Here's how the part is built. I have some questions about the finished solid (model axes, mm). A direction names the side the tool comes from. Coordinates: 2 decimals unless noted, no trailing zeros. Loops run counter-clockwise (first coordinate to the right, second up) from the corner with the lowest first, then second, coordinate; pieces in that order, holes last. Notation, with made-up numbers: (-27, -20.5) -> (-14, -20.5) arc R35 cw to (-14, 13.5) -> close; hole circle Ø1 at (-10.5, -10.5). An arc over 180 degrees is marked (long way). Answer as a JSON object with one key per item and string values. Group by question number.
1) Which directions (+Z, -Z, +X, -X, +Y, -Y) give clear straight access to the entire face, cutting with the end or side of a thin tool? Please do faces 1 (the flat face through (9.413, -7.048, 2.465)), 2 (the flat face through (3.94, 4.16, 5.07)), 3 (the flat face through (4.1, -6, 2.5)).
2) I want a section at A-A (y = 3.75). Write out the boundary of the cut face in (x, z), then the cut area to 3 significant figures.
3) If we mould it in two halves opening along Z, with no side actions, what happens to faces 4 (the cylindrical face through (4.264, -4.222, 6.479)), 5 (the cylindrical face through (5.99, 5.3, 2.46)), 6 (the flat face through (2, -4, 10))? For each: +Z half, -Z half, draft (parallel to the pull), parting line (faces both ways), or undercut.
4) I need wall thicknesses on probe 1 along Y at (x, z) = (3, 7.75); probe 2 along Z at (x, y) = (0.25, -16.25); probe 3 along X at (y, z) = (-6.75, 3). Which ranges of each line are inside material? Lowest first, please. Write a range as [from, to].
5) I'm going to push flat-ended pins straight in: pin 1 (0.5 mm diameter, centred on x = -4, y = -4, fed in from -Z); pin 2 (4 mm diameter, centred on x = 6, z = 8.5, fed in from +Y); pin 3 (2.5 mm diameter, centred on y = -8, z = 3.5, fed in from -X). Where does each tip first touch, or does it pass through?
6) I want a section at B-B (x = 9.25). Write out the boundary of the cut face in (y, z).
```python
from build123d import *

# Parameters (mm, degrees)
P_IDAT_VYSUNUT_M1_DEPTH  = 5
SKICA2_R                 = 6
SKICA2_R_2               = 4.25
P_IDAT_VYSUNUT_M2_DEPTH  = 3
SKICA3_R                 = 7.399081898
SKICA3_R_2               = 4.25
P_IDAT_VYSUNUT_M3_DEPTH  = 2
ODEBRAT_VYSUNUT_M1_DEPTH = 12
SKICA5_R                 = 0.75
ODEBRAT_VYSUNUT_M2_DEPTH = 22
ODEBRAT_VYSUNUT_M3_DEPTH = 22
ZAOBLIT1_R               = 3
ZAOBLIT2_R               = 1


with BuildPart() as part:
    # Skica1 → Přidat vysunutím1 (new body)
    with BuildSketch(Plane.XY):
        with BuildLine():
            ThreePointArc((4.25, 0), (1.26615959, -4.057011202), (-3.495571714, -2.417328772))
            Line((-3.495571714, -2.417328772), (-3.495571714, -22.417328772))
            Line((-3.495571714, -22.417328772), (2.504428286, -17.65904484))
            Line((2.504428286, -17.65904484), (2.504428286, -7.266994767))
            Line((2.504428286, -7.266994767), (6.852381906, -3.818861792))
            Line((6.852381906, -3.818861792), (11.911787503, -10.198563806))
            Line((11.911787503, -10.198563806), (15.829382947, -7.09172523))
            Line((15.829382947, -7.09172523), (6.421160578, 4.771655566))
            ThreePointArc((6.421160578, 4.771655566), (5.746609385, 5.565651855), (4.974594852, 6.26525387))
            Line((4.974594852, 6.26525387), (1.66035906, 3.912250988))
            ThreePointArc((1.66035906, 3.912250988), (3.543940322, 2.345844623), (4.25, 0))
        make_face()
    extrude(amount=P_IDAT_VYSUNUT_M1_DEPTH)

    # Skica2 → Přidat vysunutím2 (add)
    with BuildSketch(Plane.XY.offset(5)):
        with Locations(Location((0, 0, 0), (0, 0, 234.366710991))):
            Circle(SKICA2_R)
        with Locations(Location((0, 0, 0), (0, 0, 214.665420921))):
            Circle(SKICA2_R_2, mode=Mode.SUBTRACT)
    extrude(amount=P_IDAT_VYSUNUT_M2_DEPTH)

    # Skica3 → Přidat vysunutím3 (add)
    with BuildSketch(Plane.XY.offset(8)):
        Circle(SKICA3_R)
        with Locations(Location((0, 0, 0), (0, 0, 214.665420921))):
            Circle(SKICA3_R_2, mode=Mode.SUBTRACT)
    extrude(amount=P_IDAT_VYSUNUT_M3_DEPTH)

    # Skica4 → Odebrat vysunutím1 (cut)
    with BuildSketch(Plane.XY.offset(10)):
        Polygon((7.922687554, 8.36122904), (-6.923828501, -7.307080525), (-16.64765112, 7.717248389), align=None)
    extrude(amount=-ODEBRAT_VYSUNUT_M1_DEPTH, mode=Mode.SUBTRACT)

    # Skica5 → Odebrat vysunutím2 (cut)
    with BuildSketch(Plane(origin=(6.265061416, 4.968490178, 0), x_dir=(0, 0, -1), z_dir=(0.7835190888567162, 0.6213677151229708, 0))):
        with Locations(Location((-2.5, -12.392369605, 0), (0, 0, 90))):
            Circle(SKICA5_R)
    extrude(amount=-ODEBRAT_VYSUNUT_M2_DEPTH, mode=Mode.SUBTRACT)

    # Skica7 → Odebrat vysunutím3 (cut)
    with BuildSketch(Plane.XY.offset(5)):
        with BuildLine():
            Line((-3.495571714, -22.417328772), (1.368531431, -18.559864799))
            ThreePointArc((1.368531431, -18.559864799), (-1.800885961, -18.910447054), (-3.495571714, -16.209307532))
            Line((-3.495571714, -16.209307532), (-3.495571714, -22.417328772))
        make_face()
    extrude(amount=-ODEBRAT_VYSUNUT_M3_DEPTH, mode=Mode.SUBTRACT)

    # Zaoblit1
    zaoblit1_edges = [part.edges().sort_by_distance(p)[0] for p in [
        (6.852381906, -3.818861792, 2.5),
        (2.504428286, -7.266994767, 2.5),
    ]]
    fillet(zaoblit1_edges, radius=ZAOBLIT1_R)

    # Zaoblit2
    zaoblit2_edges = [part.edges().sort_by_distance(p)[0] for p in [
        (15.829382947, -7.09172523, 2.5),
        (11.911787503, -10.198563806, 2.5),
    ]]
    fillet(zaoblit2_edges, radius=ZAOBLIT2_R)


solid = part.part
```
Determined:
{
 "1": {"face 1": "+Z, -Z, -Y", "face 2": "+Z, -Z, -X, +Y", "face 3": "-Z, -Y"},
 "2": {"outline": "(3.55, 0) -> (7.23, 0) -> (7.23, 5) -> (4.68, 5) -> (4.68, 8) -> (6.38, 8) -> (6.38, 10) -> (3.55, 10) -> close", "area": "27.4 mm^2"},
 "3": {"face 4": "undercut", "face 5": "draft", "face 6": "+Z half"},
 "4": {"probe 1": "[-5.2, -3.01], [3.01, 3.17]", "probe 2": "[0, 1.94], [3.06, 5]", "probe 3": "[-3.5, 3.24], [9.18, 10.53], [12.33, 15.41]"},
 "5": {"pin 1": "z = 5", "pin 2": "y = 5.37", "pin 3": "x = -3.5"},
 "6": {"outline": "(-6.84, 0) -> (1.2, 0) -> (1.2, 5) -> (-6.84, 5) -> close"}
}
